Autodesk Inventor part; units mm, degrees
ref_plane "YZ Plane" through (0, 0, 0) normal (1, 0, 0) x (0, 1, 0)
ref_plane "XZ Plane" through (0, 0, 0) normal (0, 1, 0) x (-1, 0, 0)
ref_plane "XY Plane" through (0, 0, 0) normal (0, 0, 1) x (1, 0, 0)
ref_plane "Arbeitsebene1" through (426.5914, 236.3923, -168.6308) normal (0, 0, -1) x (0.9998, 0.0217, 0)
sketch "Skizze1" plane through (426.5914, 236.3923, -168.6308) normal (0, 0, -1) x (0.9998, 0.0217, 0)
  circle A0 centre (-10, -17.5) radius 1.4
  arc A1 (-22.2323, -12) -> (-21.7536, -14.2401) centre (-19.0971, -12.5012) ccw
  arc A2 (-21.7536, -14.2401) -> (-13.215, -22.3912) centre (0, 0) ccw
  arc A3 (-13.215, -22.3912) -> (-8.8966, -21.32) centre (-11.6012, -19.6569) ccw
  arc A4 (-2.8797, -22.9216) -> (-8.8966, -21.32) centre (-6.1282, -23.0224) ccw
  arc A5 (-2.8797, -22.9216) -> (0.3346, -25.9978) centre (0.2937, -22.8231) ccw
  arc A6 (0.3346, -25.9978) -> (25.1076, -6.7536) centre (0, 0) ccw
  arc A7 (25.1076, -6.7536) -> (24.1419, -5.4938) centre (24.1419, -6.4938) ccw
  line L0 (24.1419, -5.4938) -> (21.5, -5.4938)
  arc A8 (21.5, -5.4938) -> (20.5, -6.4938) centre (21.5, -6.4938) ccw
  line L1 (20.5, -6.4938) -> (20.5, -12.25)
  arc A9 (19.5653, -13.9427) -> (20.5, -12.25) centre (18.5, -12.25) ccw
  arc A10 (19.5653, -13.9427) -> (18.3317, -15.4908) centre (21.1633, -16.4816) ccw
  arc A11 (15.5, -17.5) -> (18.3317, -15.4908) centre (15.5, -14.5) ccw
  line L2 (15.5, -17.5) -> (11.4, -17.5)
  arc A12 (10.611, -16.2403) -> (11.4, -17.5) centre (10, -17.5) ccw
  line L3 (10.611, -16.2403) -> (10.611, -14.3079)
  arc A13 (10.611, -14.3079) -> (10.0242, -14.25) centre (10.0242, -17.25) ccw
  line L4 (10.0242, -14.25) -> (-18.5, -14.25)
  arc A14 (-20.5, -12.25) -> (-18.5, -14.25) centre (-18.5, -12.25) ccw
  line L5 (-20.5, -12.25) -> (-20.5, -12)
  line L6 (-22.2323, -12) -> (-20.5, -12)
  arc A15 (14.1536, 17.8908) -> (13.1449, 22.4324) centre (11.5397, 19.693) ccw
  arc A16 (13.1449, 22.4324) -> (-23.0651, 12) centre (0, 0) ccw
  line L7 (-20.5, 12) -> (-23.0651, 12)
  line L8 (-20.5, 12) -> (-20.5, 12.25)
  arc A17 (-18.5, 14.25) -> (-20.5, 12.25) centre (-18.5, 12.25) ccw
  line L9 (-18.5, 14.25) -> (10.0242, 14.25)
  arc A18 (10.0242, 14.25) -> (10.611, 14.3079) centre (10.0242, 17.25) ccw
  line L10 (10.611, 14.3079) -> (10.611, 16.2403)
  arc A19 (11.3618, 17.8248) -> (10.611, 16.2403) centre (10, 17.5) ccw
  line L11 (11.3618, 17.8248) -> (14.1093, 17.8248)
  arc A20 (14.1536, 17.8908) -> (14.1093, 17.8248) centre (16.8293, 16.046) ccw
  circle A21 centre (-10, 17.5) radius 1.4
  circle A22 centre (10, 17.5) radius 1.4
  circle A23 centre (10, -17.5) radius 1.4
  circle A24 centre (0, 0) radius 26
  circle A25 centre (0, 0) radius 24.1513
  line L12 (-20.5, -12) -> (-20.5, 12)
  arc A26 (23.033, 12.0616) -> (19.834, 13.7401) centre (20.2203, 10.5887) ccw
  arc A27 (20.5, 12.25) -> (19.834, 13.7401) centre (18.5, 12.25) ccw
  line L13 (20.5, 12.25) -> (20.5, 7.4938)
  arc A28 (20.5, 7.4938) -> (21.5, 6.4938) centre (21.5, 7.4938) ccw
  line L14 (21.5, 6.4938) -> (23.8504, 6.4938)
  arc A29 (23.8504, 6.4938) -> (24.8044, 7.7936) centre (23.8504, 7.4938) ccw
  arc A30 (24.8044, 7.7936) -> (23.033, 12.0616) centre (0, 0) ccw
  line L15 (20.5, -6.4938) -> (20.5, 7.4938)
  line L16 (10.611, 14.3079) -> (19.4569, 14.3079)
  line L17 (10.0242, -14.25) -> (19.4993, -14.25)
  point P0 (-431.6269, 227.0676)
  point P1 (14.6734, 19.1827)
  point P2 (19.9142, 13.6642)
  point P3 (19.9142, -13.6642)
  point P4 (18.1109, -15.9775)
  point P5 (13.1449, 22.4324)
  point P6 (-21.7536, -14.2401)
  point P7 (-13.215, -22.3912)
  point P8 (0.3346, -25.9978)
  point P9 (25.1076, -6.7536)
  point P10 (11.4, -17.5)
extrude "Extrusion1" add sketch "Skizze1" along normal blind 8 contours L6 A25 A14 A3 A2 A1 | A1 A24 L7 A25 L6 | A25 L7 L12 L6 | L6 L5 A14 A25 | A3 A25 A5 A24 | A16 A15 A25 A17 L7 | L17 A10 A11 A25 L2 A23 L3 A13 | A25 A17 L8 L7 | A25 A14 L4 A13 L3 A12 L2 A11 A5 A4 A3 | A3 A4 A5 A25 | A5 A25 A11 A9 L0 A7 A6 | A24 A26 A25 A15 | A7 L0 A25 L14 A29 A24 | A25 L16 L10 A22 L11 A20 A15 | A15 A20 L11 A19 L10 A18 L9 A17 A25 | A24 A29 L14 A25 A27 A26 | A25 A11 | A11 A10 L17 A25 | A25 A9 L1 A8 L0 | L0 A8 L15 A28 L14 A25 | L14 A28 L13 A27 A25
properties part number "Anglerfish_spacer8mm_bottom_v0"
Geometry: final body of the model. Coordinates: model frame, mm. A direction names the side the tool comes from. Give positions to 0.01 mm unless a question says otherwise; leave off trailing zeros. Loops run counter-clockwise (first coordinate to the right, second up) from the corner with the lowest first, then second, coordinate; pieces in that order, holes last. Notation, with made-up numbers: M 76.25,-11 L 101.25,-11 A28 ccw 101.25,22 Z; hole C 13,63 d10. An arc over 180 degrees is marked long. Put each result on its own line as item: value.
1) Cut plane C-C, the plane z = -170. Return the cut outline in (x, y), plus the area to 3 significant figures.
Computed values:
outline: M 403.79,223.89 A26 ccw 440.22,214.25 A26 ccw 451.55,243.69 A26 ccw 426.36,262.39 A26 ccw 412.89,258.49 A26 ccw 404.53,250.16 A26 ccw Z; hole M 405.83,248.19 L 406.36,223.7 A2 ccw 408.4,221.74 L 436.92,222.36 A3 cw 437.51,222.32 L 446.35,222.51 A24.15 ccw 446.8,223.16 A2 ccw 447.35,224.59 L 446.82,249.08 A2 ccw 446.2,250.49 A24.15 ccw 445.78,251.06 L 407.79,250.24 A2 ccw Z; hole C 416.21,253.67 d2.8; hole C 416.97,218.68 d2.8; hole M 436.85,252.86 A1.4 ccw 437.61,254.14 A1.4 ccw long Z; hole M 437.55,220.39 A1.4 ccw long 438.34,218.82 A1.4 ccw Z
area: 933 mm^2
2) Mould query, pull axis Y, two halves, no side actions, for faces 3 (the cylindrical face through (435.034, 254.865, -172.575)), 4 (the cylindrical face through (419.455, 261.394, -172.575)), 5 (the cylindrical face through (400.608, 237.319, -172.575)). Classes: released by +Y, released by -Y, zero draft, split by the parting line, or undercut.
Computed values:
face 3: undercut
face 4: released by +Y
face 5: split by the parting line
3) Material intervals for L1, parallel to Y at x = 416.5, z = -170.5; L2, parallel to Y at x = 408.5, z = -173.75; L3, parallel to X at y = 219, z = -172.75, sorted ascending. Write a range as from..to.
Computed values:
L1: y = 212.43..217.36, 220..221.92, 250.43..252.3, 255.04..260.35
L2: y = 217.72..221.75, 250.25..255.07
L3: x = 407.27..415.61, 418.34..435.57, 438.36..445.92
4) Cut plane B-B, the plane x = 409. Return the cut outline in (y, z).
Computed values:
outline: M 217.25,-176.63 L 221.76,-176.63 L 221.76,-168.63 L 217.25,-168.63 Z; M 250.26,-176.63 L 255.54,-176.63 L 255.54,-168.63 L 250.26,-168.63 Z
5) Cut plane D-D, the plane x = 416.5. Return the cut outline in (y, z), plus the area to 3 significant figures.
Computed values:
outline: M 212.43,-176.63 L 217.36,-176.63 L 217.36,-168.63 L 212.43,-168.63 Z; M 220,-176.63 L 221.92,-176.63 L 221.92,-168.63 L 220,-168.63 Z; M 250.43,-176.63 L 252.3,-176.63 L 252.3,-168.63 L 250.43,-168.63 Z; M 255.04,-176.63 L 260.35,-176.63 L 260.35,-168.63 L 255.04,-168.63 Z
area: 112 mm^2
6) First-contact query: P1, Ø2, axis at x = 425.5, z = -173, coming from the +Y side; P2, Ø1.5, axis at y = 240, z = -173.5, coming from the -X side. Flat tips, straight axial feed; report the tip coordinate or a pass-through.
Computed values:
P1: stops at y = 262.39
P2: stops at x = 400.75
7) Cut plane A-A, the plane y = 234.5. Return the cut outline in (x, z), plus the area to 3 significant figures.
Computed values:
outline: M 400.66,-176.63 L 406.13,-176.63 L 406.13,-168.63 L 400.66,-168.63 Z; M 447.14,-176.63 L 452.52,-176.63 L 452.52,-168.63 L 447.14,-168.63 Z
area: 86.8 mm^2
8) Reachability of faces 1 (the flat face through (428, 252, -168.631)), 2 (the cylindrical face through (447.213, 223.811, -172.575)) from +Z, -Z, +X, -X, +Y, -Y: full face, straight path, thin tool, end or side. Return the list, or none.
Computed values:
face 1: +Z, +X, -X, +Y, -Y
face 2: +Z, -Z
